Verification items for the finished model (mm, model axes). A direction names the side the tool comes from. Coordinates: 2 decimals unless noted, no trailing zeros. Order: outer loops, then holes, each group sorted by start corner. A loop starts at its lowest first (then second) coordinate and runs counter-clockwise, first axis right, second up. Notation, with made-up numbers: (45.5, 32) - (95.5, 32) arc R22 cw to (95.5, 44) - close; hole circle Ø9 at (75.5, 28.25). An arc over 180 degrees is marked (long way). Answer as CSV lines item,"result". Start each with the question number.
1. Go/stop test with flat-tipped pins: pin 1 (12 mm diameter, centred on x = -5, y = 6, fed in from +Z); pin 2 (8 mm diameter, centred on x = -6.5, z = -33.5, fed in from +Y) (3 decimals); pin 3 (8 mm diameter, centred on x = 6, z = -33.5, fed in from -Y). Record where each tip stops, or that it passes through.
2. Section check C-C (y = -18). Record the cut outline in (x, z).
3. Set-up check for faces 4 (the flat face through (-8, -15, -21)), 5 (the flat face through (11, -16, -12)), 6 (the flat face through (11.042, -15.88, -27.745)): record each of +Z, -Z, +X, -X, +Y, -Y from which the full face is reachable in a straight line by a thin tool's end or side.
4. Mould release check, pull along X, two halves, no side actions. Record for faces 1 (the flat face through (-11, -16, -12)), 2 (the flat face through (8, -16, 4)), 3 (the flat face through (-14, -9, -8)): pulls with the +X half, pulls with the -X half, needs draft (parallel to the pull), parting line crosses it, or undercut.
5. Section check B-B (y = -28). Record the cut outline in (x, z).
6. Section check A-A (z = 9). Record the cut outline in (x, y).
7. Section check D-D (x = 0). Record the cut outline in (y, z), and give its area (3 significant figures).
8. Material ranges on L1, parallel to Z at x = 12.5, y = -18; L2, parallel to Z at x = 10, y = -19.5 (3 decimals); L3, parallel to Y at x = -0.5, z = -13, recorded low to high. Write a range as [from, to].
from build123d import *

# Parameters (mm, degrees)
SKETCH1_R               = 14
BOSS_EXTRUDE1_DEPTH     = 50
SKETCH2_R               = 3.5
SKETCH2_R_2             = 2.5
BOSS_EXTRUDE2_DEPTH     = 14
CUT_EXTRUDE3_DEPTH      = 61.834364638
CUT_EXTRUDE3_DEPTH_BACK = 61.834364638
CUT_EXTRUDE4_START      = 57
CUT_EXTRUDE4_DEPTH      = 57
SKETCH6_R               = 11
CUT_EXTRUDE5_DEPTH      = 40


with BuildPart() as part:
    # Sketch1 → Boss-Extrude1 (new body)
    with BuildSketch(Plane.XY):
        Circle(SKETCH1_R)
    extrude(amount=-BOSS_EXTRUDE1_DEPTH)

    # Sketch2 → Boss-Extrude2 (add, symmetric)
    with BuildSketch(Plane(origin=(0, 0, 0), x_dir=(0, 0, -1), z_dir=(1, 0, 0))):
        with BuildLine():
            Line((15, -24), (23.267238418, -24))
            ThreePointArc((23.267238418, -24), (25.093522705, -23.380060021), (26.165015897, -21.776457135))
            Line((26.165015897, -21.776457135), (32, 0))
            Line((32, 0), (0, 0))
            Line((0, 0), (-12.179515585, -7.61060601))
            ThreePointArc((-12.179515585, -7.61060601), (-14.903885139, -11.629249661), (-13.762573354, -16.348263718))
            Line((-13.762573354, -16.348263718), (-2, -31.698894587))
            Line((-2, -31.698894587), (0, -31.698894587))
            Line((0, -31.698894587), (0, -25.927651143))
            ThreePointArc((0, -25.927651143), (5.280940814, -19.913790946), (6.988586602, -12.094660803))
            ThreePointArc((6.988586602, -12.094660803), (9.446060431, -9.493846328), (12, -12))
            Line((12, -12), (12, -21))
            ThreePointArc((12, -21), (12.878679656, -23.121320344), (15, -24))
        make_face()
        with Locations((-9, -12.698894587)):
            Circle(SKETCH2_R, mode=Mode.SUBTRACT)
        with Locations((19.929981273, -18)):
            Circle(SKETCH2_R_2, mode=Mode.SUBTRACT)
    extrude(amount=BOSS_EXTRUDE2_DEPTH, both=True)

    # Sketch4 → Cut-Extrude3 (cut, two sides: drawn at the far end of the back side and taken through both)
    with BuildSketch(Plane.XY.offset(-CUT_EXTRUDE3_DEPTH_BACK)):
        with BuildLine():
            Line((-8, -31.698894587), (-8, -11.489125293))
            ThreePointArc((-8, -11.489125293), (0, -14), (8, -11.489125293))
            Line((8, -11.489125293), (8, -31.698894587))
            Line((8, -31.698894587), (-8, -31.698894587))
        make_face()
    extrude(amount=CUT_EXTRUDE3_DEPTH + CUT_EXTRUDE3_DEPTH_BACK, mode=Mode.SUBTRACT)

    # Sketch5 → Cut-Extrude4 (cut)
    with BuildSketch(Plane.XY.offset(CUT_EXTRUDE4_START)):
        with BuildLine():
            Line((-8, 0), (8, 0))
            Line((8, 0), (8, -11.489125293))
            ThreePointArc((8, -11.489125293), (0, -14), (-8, -11.489125293))
            Line((-8, -11.489125293), (-8, 0))
        make_face()
    extrude(amount=-CUT_EXTRUDE4_DEPTH, mode=Mode.SUBTRACT)

    # Sketch6 → Cut-Extrude5 (cut)
    with BuildSketch(Plane(origin=(0, 0, -50), x_dir=(-1, 0, 0), z_dir=(0, 0, -1))):
        Circle(SKETCH6_R)
    extrude(amount=-CUT_EXTRUDE5_DEPTH, mode=Mode.SUBTRACT)


solid = part.part
Evaluation:
1,pin 1,"stops at z = 0"
1,pin 2,"stops at y = 13.775"
1,pin 3,"stops at y = -13.86"
2,outline,"(-14, -27.18) - (-8, -27.18) - (-8, -22.43) - (-14, -22.43) - close; (-14, -17.43) - (-8, -17.43) - (-8, -12) - (-14, -12) - close; (-14, -6.1) - (-8, -6.1) - (-8, 12.5) - (-14, 12.5) - close; (8, -27.18) - (14, -27.18) - (14, -22.43) - (8, -22.43) - close; (8, -17.43) - (14, -17.43) - (14, -12) - (8, -12) - close; (8, -6.1) - (14, -6.1) - (14, 12.5) - (8, 12.5) - close"
3,face 4,"+Z, -Z, -Y"
3,face 5,"+X, -Y"
3,face 6,"-Z, +X, -Y"
4,face 1,"needs draft"
4,face 2,"undercut"
4,face 3,"pulls with the -X half"
5,outline,"(-14, 0) - (-8, 0) - (-8, 4.83) - (-14, 4.83) - close; (8, 0) - (14, 0) - (14, 4.83) - (8, 4.83) - close"
6,outline,"(-14, -22.56) - (-8, -22.56) - (-8, -16.2) - (-14, -16.2) - close; (-14, -9.2) - (-8, -9.2) - (-8, -5.62) - (-14, -5.62) - close; (8, -22.56) - (14, -22.56) - (14, -16.2) - (8, -16.2) - close; (8, -9.2) - (14, -9.2) - (14, -5.62) - (8, -5.62) - close"
7,outline,"(-14, -50) - (-11, -50) - (-11, -10) - (11, -10) - (11, -50) - (14, -50) - (14, 0) - (-14, 0) - close"
7,area,"520 mm²"
8,L1,"z = [-27.18, -22.43], [-17.43, -12], [-6.1, 12.5]"
8,L2,"z = [-26.775, -21.93], [-17.93, -12], [-5.483, 11.348]"
8,L3,"y = [-13.99, -10.99], [10.99, 13.99]"
